The model under review builds one solid part; all positions refer to its coordinate system, in mm. A direction names the side the tool comes from. Coordinates: 2 decimals unless noted, no trailing zeros. Loops run counter-clockwise (first coordinate to the right, second up) from the corner with the lowest first, then second, coordinate; pieces in that order, holes last. Notation, with made-up numbers: M 28,46 L 34,46 A20 ccw 34,51 Z; hole C 75.25,-34 d7. An arc over 180 degrees is marked long. Use one line per item in the form item = value.
```python
from build123d import *

# Parameters (mm, degrees)
F0_W      = 63
F0_H      = 75
F1_DEPTH  = 75
F2_W      = 38
F2_H      = 35
F3_DEPTH  = 75
F4_W      = 19
F4_H      = 67
F5_DEPTH  = 45
F7_DEPTH  = 28
F9_DEPTH  = 25
F11_DEPTH = 19
F13_DEPTH = 19
F15_DEPTH = 100


with BuildPart() as f1:
    # F0 (on Top) → F1 (new body)
    with BuildSketch(Plane.XY):
        with Locations((-19.216308, -1.011902)):
            Rectangle(F0_W, F0_H)
    extrude(amount=F1_DEPTH)

    # F2 (on face) → F3 (cut)
    with BuildSketch(Plane.XZ.offset(38.511902)):
        with Locations((-31.716308, 37.5)):
            Rectangle(F2_W, F2_H)
    extrude(amount=-F3_DEPTH, mode=Mode.SUBTRACT)

    # F4 (on face) → F5 (join)
    with BuildSketch(Plane.YZ.offset(12.283692)):
        with Locations((-21.011902, 33.5)):
            Rectangle(F4_W, F4_H)
        with Locations((18.988098, 33.5)):
            Rectangle(F4_W, F4_H)
    extrude(amount=F5_DEPTH)

    # F6 (on face) → F7 (join)
    with BuildSketch(Plane.YZ.offset(12.283692)):
        Polygon((-11.511902, 75), (-11.511902, 67), (-11.511902, 0), (9.488098, 0), (9.488098, 67), (9.488098, 75), align=None)
    extrude(amount=F7_DEPTH)

    # F8 (on face) → F9 (cut)
    with BuildSketch(Plane.XZ.offset(11.511902)):
        Polygon((40.283692, 75), (12.283692, 75), (40.283692, 67), align=None)
    extrude(amount=-F9_DEPTH, mode=Mode.SUBTRACT)

    # F10 (on face) → F11 (join)
    with BuildSketch(Plane.XZ.offset(30.511902)):
        with BuildLine():
            Line((57.283692, 67), (57.283692, 0))
            ThreePointArc((57.283692, 0), (90.783692, 33.5), (57.283692, 67))
        make_face()
    extrude(amount=-F11_DEPTH)

    # F12 (on face) → F13 (join)
    with BuildSketch(Plane(origin=(0, 28.488098, 0), x_dir=(-1, 0, 0), z_dir=(0, 1, 0))):
        with BuildLine():
            Line((-57.283692, 0), (-57.283692, 67))
            ThreePointArc((-57.283692, 67), (-90.783692, 33.5), (-57.283692, 0))
        make_face()
    extrude(amount=-F13_DEPTH)

    # F14 (on face) → F15 (cut)
    with BuildSketch(Plane.XZ.offset(30.511902)):
        with BuildLine():
            ThreePointArc((69.783692, 33.5), (66.122527, 42.338835), (57.283692, 46))
            ThreePointArc((57.283692, 46), (48.444857, 24.661165), (69.783692, 33.5))
        make_face()
    extrude(amount=-F15_DEPTH, mode=Mode.SUBTRACT)


solid = f1.part
```
1. Insertion check: P1, Ø15, axis at x = 57.28, z = 33.5, coming from the -Y side; P2, Ø1, axis at x = 39, z = 27.5, coming from the +Y side; P3, Ø2.5, axis at x = 33, z = 69.5, coming from the +Y side; P4, Ø12, axis at x = 26, z = 41.5, coming from the -Y side. Each pin has a flat end and moves straight along its axis. Give the tip position at first contact, or say it passes through.
Response values:
P1 = through
P2 = 28.49
P3 = 9.49
P4 = -30.51
2. Add section D-D (y = -9). State the section outline as (x, z) points.
Response values:
outline = M -50.72,0 L 40.28,0 L 40.28,67 L 12.28,75 L -50.72,75 L -50.72,55 L -12.72,55 L -12.72,20 L -50.72,20 Z
3. Add section B-B (z = 28). State the section outline as (x, y) points.
Response values:
outline = M -12.72,-38.51 L 12.28,-38.51 L 12.28,-30.51 L 46.06,-30.51 L 46.06,-11.51 L 40.28,-11.51 L 40.28,9.49 L 46.06,9.49 L 46.06,28.49 L 12.28,28.49 L 12.28,36.49 L -12.72,36.49 Z; M 68.51,-30.51 L 90.33,-30.51 L 90.33,-11.51 L 68.51,-11.51 Z; M 68.51,9.49 L 90.33,9.49 L 90.33,28.49 L 68.51,28.49 Z
4. Machinability: for faces 1 (the face through (-32, -2, 55)), 2 (the face through (43, 28.488, 34)), 3 (the face through (71, -11.512, 34)), 4 (the face through (34, 19, 67)), which of the approach directions +Z, -Z, +X, -X, +Y, -Y give a long, thin tool a straight path to every point of the face, cutting with its end or side? Answer none if there is none.
Response values:
face_1 = -X, +Y, -Y
face_2 = +Z, -Z, +X, +Y
face_3 = +Z, -Z, +X
face_4 = +Z, +X, +Y
5. Add section C-C (x = 59). State the section outline as (y, z) points, then the cut area to 3 significant figures.
Response values:
outline = M -30.51,0.04 L -11.51,0.04 L -11.51,21.12 L -30.51,21.12 Z; M -30.51,45.88 L -11.51,45.88 L -11.51,66.96 L -30.51,66.96 Z; M 9.49,0.04 L 28.49,0.04 L 28.49,21.12 L 9.49,21.12 Z; M 9.49,45.88 L 28.49,45.88 L 28.49,66.96 L 9.49,66.96 Z
area = 1,600 mm^2
6. The part is to be moulded in two halves that separate along Y. For faces 5 (the face through (20, -11.512, 69)), 6 (the face through (71, 9.488, 34)), 7 (the face through (-12.716, -2, 37)), say which applies: pulls with the +Y half, pulls with the -Y half, needs draft (parallel to the pull), parting line crosses it, or undercut.
Response values:
face_5 = pulls with the -Y half
face_6 = undercut
face_7 = needs draft
7. Add section A-A (y = -26). State the section outline as (x, z) points, then the cut area to 3 significant figures.
Response values:
outline = M -50.72,0 L 57.28,0 A33.5 ccw 57.28,67 L 12.28,67 L 12.28,75 L -50.72,75 L -50.72,55 L -12.72,55 L -12.72,20 L -50.72,20 Z; hole C 57.28,33.5 d25
area = 7,680 mm^2
8. Wall thickness on line 1 along X through (y, z) = (-21, 33.5); line 2 along Y through (x, z) = (79, 54.5); line 3 along Z through (x, y) = (26.5, 24): over which ranges is each line inside the solid? List them lowest first. Write a range as from..to.
Response values:
line_1 = -12.72..44.78, 69.78..90.78
line_2 = -30.51..-11.51, 9.49..28.49
line_3 = 0..67
